Work out the finished part from the listing and answer in its coordinate system (mm). Face numbers are marked on the shaded views. Coordinates: 2 decimals unless noted, no trailing zeros. Order: outer loops, then holes, each group sorted by start corner. A loop starts at its lowest first (then second) coordinate and runs counter-clockwise, first axis right, second up. Notation, with made-up numbers: M 6.25,63 L 15.25,63 A18 cw 15.25,82 Z; hole C 63,71.25 d4. An arc over 180 degrees is marked long. Answer in a Markdown table with one row per item. Add a question column.
Item 1: The part is cut by section A-A (x = -12.5). Write down the section's boundary in (y, z), then the cut area to 3 significant figures.
Item 2: Consider line 1 (Y direction, x = 27, z = 52.5); line 2 (Y direction, x = -10, z = 57.5); line 3 (Z direction, x = 6.5, y = 23). Determine where each line is inside the solid, lowest interval first. Write a range as from..to.
Item 3: The part is cut by section C-C (z = 34). Write down the section's boundary in (x, y).
Item 4: The part is cut by section D-D (x = 32.5). Write down the section's boundary in (y, z), then the cut area to 3 significant figures.
Item 5: Flat-ended cylindrical pins translate along their axes: pin 1 Ø3 at (x, z) = (27.5, 16.5) entering from -Y; pin 2 Ø4 at (y, z) = (36, 42) entering from +X; pin 3 Ø1.5 at (x, y) = (-11.5, 11.5) entering from -Z; pin 4 Ø2.5 at (y, z) = (51.5, 47.5) entering from -X. Find the tip coordinate at first contact, or state that the pin passes through.
Item 6: The part is cut by section B-B (z = 11). Write down the section's boundary in (x, y).
Item 7: The mould has two halves that part along Y. Classify the marked faces 1, 2 and 3: released by +Y, released by -Y, zero draft, split by the parting line, or undercut.
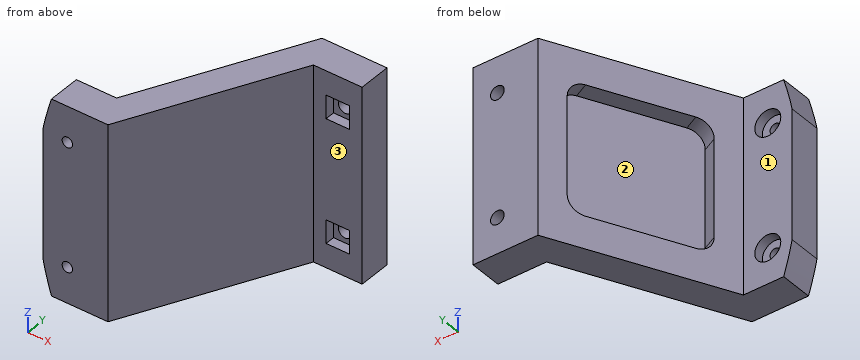
from build123d import *

# Parameters (mm, degrees)
EXTRUDE_1_DEPTH     = 60
SKETCH_2_R          = 171.976759521
SKETCH_2_R_2        = 100
CUT_EXTRUDE_1_DEPTH = 60
SKETCH_3_W          = 40
SKETCH_3_H          = 40
CUT_EXTRUDE_2_DEPTH = 5
FILLET_1_R          = 5
SKETCH_4_R          = 1.6
CUT_EXTRUDE_3_DEPTH = 10
SKETCH_5_R          = 4
CUT_EXTRUDE_4_DEPTH = 3
SKETCH_6_R          = 2.1
CUT_EXTRUDE_5_DEPTH = 88.749643874
SKETCH_7_W          = 7.2
SKETCH_7_H          = 7.2
CUT_EXTRUDE_6_DEPTH = 3


with BuildPart() as part:
    # 草图1 → 凸台-拉伸1 (new body)
    with BuildSketch(Plane.XY):
        Polygon((0, 0), (-20, 0), (-20, 10), (-5, 10), (20, 60), (40, 60), (40, 50), (25, 50), align=None)
    extrude(amount=EXTRUDE_1_DEPTH)

    # 草图2 → 切除-拉伸1 (cut)
    with BuildSketch(Plane(origin=(0, 10, 0), x_dir=(1, 0, 0), z_dir=(0, 1, 0))):
        with Locations((78, -30)):
            Circle(SKETCH_2_R)
        with Locations((78, -30)):
            Circle(SKETCH_2_R_2, mode=Mode.SUBTRACT)
    extrude(amount=-CUT_EXTRUDE_1_DEPTH, mode=Mode.SUBTRACT)

    # 草图3 → 切除-拉伸2 (cut)
    with BuildSketch(Plane(origin=(-8, 4, 0), x_dir=(0, 0, 1), z_dir=(-0.894427190999916, 0.4472135954999579, 0))):
        with Locations((30, 34.659053651)):
            Rectangle(SKETCH_3_W, SKETCH_3_H)
    extrude(amount=-CUT_EXTRUDE_2_DEPTH, mode=Mode.SUBTRACT)

    # 圆角1
    fillet_1_edges = [part.edges().sort_by_distance(p)[0] for p in [
        (18.680339887, 51.770509831, 50),
        (0.791796068, 15.993422191, 50),
        (0.791796068, 15.993422191, 10),
        (18.680339887, 51.770509831, 10),
    ]]
    fillet(fillet_1_edges, radius=FILLET_1_R)

    # 草图4 → 切除-拉伸3 (cut)
    with BuildSketch(Plane(origin=(0, 10, 0), x_dir=(1, 0, 0), z_dir=(0, 1, 0))):
        with Locations(Location((-12.5, -49, 0), (0, 0, 270))):
            Circle(SKETCH_4_R)
        with Locations(Location((-12.5, -11, 0), (0, 0, 270))):
            Circle(SKETCH_4_R)
    extrude(amount=-CUT_EXTRUDE_3_DEPTH, mode=Mode.SUBTRACT)

    # 草图5 → 切除-拉伸4 (cut)
    with BuildSketch(Plane(origin=(0, 10, 0), x_dir=(1, 0, 0), z_dir=(0, 1, 0))):
        with Locations(Location((-12.5, -49, 0), (0, 0, 270))):
            Circle(SKETCH_5_R)
        with Locations(Location((-12.5, -11, 0), (0, 0, 270))):
            Circle(SKETCH_5_R)
    extrude(amount=-CUT_EXTRUDE_4_DEPTH, mode=Mode.SUBTRACT)

    # 草图6 → 切除-拉伸5 (cut, through all)
    with BuildSketch(Plane.XZ.offset(-50)):
        with Locations(Location((32.5, 11, 0), (0, 0, 270))):
            Circle(SKETCH_6_R)
        with Locations(Location((32.5, 49, 0), (0, 0, 270))):
            Circle(SKETCH_6_R)
    extrude(amount=-CUT_EXTRUDE_5_DEPTH, mode=Mode.SUBTRACT)

    # 草图7 → 切除-拉伸6 (cut)
    with BuildSketch(Plane.XZ.offset(-50)):
        with Locations((32.5, 11)):
            Rectangle(SKETCH_7_W, SKETCH_7_H)
        with Locations((32.5, 49)):
            Rectangle(SKETCH_7_W, SKETCH_7_H)
    extrude(amount=-CUT_EXTRUDE_6_DEPTH, mode=Mode.SUBTRACT)


solid = part.part
Reply:
| question | item | result |
|---|---|---|
| 1 | outline | M 0,0 L 10,0 L 10,7 L 7,7 L 7,9.4 L 0,9.4 Z; M 0,12.6 L 7,12.6 L 7,15 L 10,15 L 10,45 L 7,45 L 7,47.4 L 0,47.4 Z; M 0,50.6 L 7,50.6 L 7,53 L 10,53 L 10,60 L 0,60 Z |
| 1 | area | 507 mm2 |
| 2 | line 1 | y = 50..60 |
| 2 | line 2 | y = 0..10 |
| 2 | line 3 | z = 0..10, 50..60 |
| 3 | outline | M -20,0 L 0,0 L 25,50 L 40,50 L 40,60 L 20,60 L 16.44,52.89 L 20.92,50.65 L 3.03,14.88 L -1.44,17.11 L -5,10 L -20,10 Z |
| 4 | outline | M 50,0 L 60,0 L 60,8.9 L 53,8.9 L 53,7.4 L 50,7.4 Z; M 50,14.6 L 53,14.6 L 53,13.1 L 60,13.1 L 60,46.9 L 53,46.9 L 53,45.4 L 50,45.4 Z; M 50,52.6 L 53,52.6 L 53,51.1 L 60,51.1 L 60,60 L 50,60 Z |
| 4 | area | 498 mm2 |
| 5 | pin 1 | stops at y = 50 |
| 5 | pin 2 | stops at x = 19 |
| 5 | pin 3 | passes through |
| 5 | pin 4 | stops at x = 15.69 |
| 6 | outline | M -20,0 L -14.1,0 L -14.1,7 L -16.5,7 L -16.5,10 L -20,10 Z; M -10.9,0 L 0,0 L 25,50 L 28.9,50 L 28.9,53 L 30.4,53 L 30.4,60 L 20,60 L 15.55,51.1 L 20.02,48.86 L 3.92,16.66 L -0.55,18.9 L -5,10 L -8.5,10 L -8.5,7 L -10.9,7 Z; M 34.6,53 L 36.1,53 L 36.1,50 L 40,50 L 40,60 L 34.6,60 Z |
| 7 | face 1 | released by +Y |
| 7 | face 2 | undercut |
| 7 | face 3 | released by -Y |
